Part print with two shaded views. Sizes in mm from the minimum x, y, z corner. Round coordinates to 2 decimals unless told otherwise and drop trailing zeros. Order: outer loops, then holes, each group sorted by start corner. A loop starts at its lowest first (then second) coordinate and runs counter-clockwise, first axis right, second up. Notation, with made-up numbers: (73, 85.5) -> (81, 85.5) arc R11 ccw to (81, 100.5) -> close; hole circle Ø7 at (-7, 44.25). An arc over 180 degrees is marked (long way). Use a Markdown table: item, result. Add a question column.
Item 1: Slice it at B-B, the plane z = 97. Give the cut face in (x, y).
Item 2: Slice it at C-C, the plane x = 81.5. Give the cut face in (y, z).
Item 3: Pin check, flat tip, straight feed: pin 1 (2.5 mm diameter, centred on x = 5, z = 2.5, fed in from -Y). Stop position of the tip, or through.
Item 4: Slice it at A-A, the plane y = 160.5. Give the cut face in (x, z), plus the area to 3 significant figures.
Item 5: Probe L1, parallel to Z at x = 10, y = 128; L2, parallel to Y at x = 114.5, z = 189. List the from-to ranges inside material, lowest first.
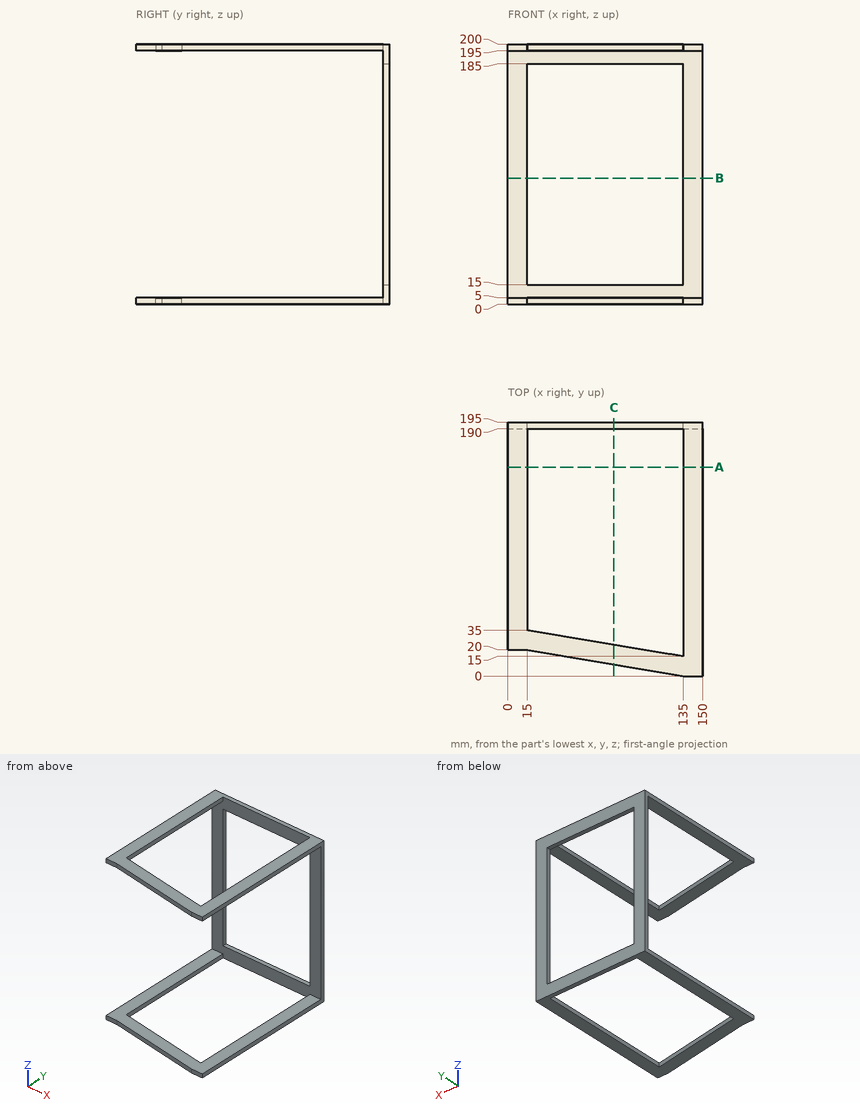
Check sheet entries:
| question | item | result |
|---|---|---|
| 1 | outline | (0, 190) -> (15, 190) -> (15, 195) -> (0, 195) -> close; (135, 190) -> (150, 190) -> (150, 195) -> (135, 195) -> close |
| 2 | outline | (8.92, 0) -> (23.92, 0) -> (23.92, 5) -> (8.92, 5) -> close; (8.92, 195) -> (23.92, 195) -> (23.92, 200) -> (8.92, 200) -> close; (190, 0) -> (195, 0) -> (195, 15) -> (190, 15) -> close; (190, 185) -> (195, 185) -> (195, 200) -> (190, 200) -> close |
| 3 | pin 1 | y = 20 |
| 4 | outline | (0, 0) -> (15, 0) -> (15, 5) -> (0, 5) -> close; (0, 195) -> (15, 195) -> (15, 200) -> (0, 200) -> close; (135, 0) -> (150, 0) -> (150, 5) -> (135, 5) -> close; (135, 195) -> (150, 195) -> (150, 200) -> (135, 200) -> close |
| 4 | area | 300 mm2 |
| 5 | L1 | 0 to 5, 195 to 200 |
| 5 | L2 | 190 to 195 |
